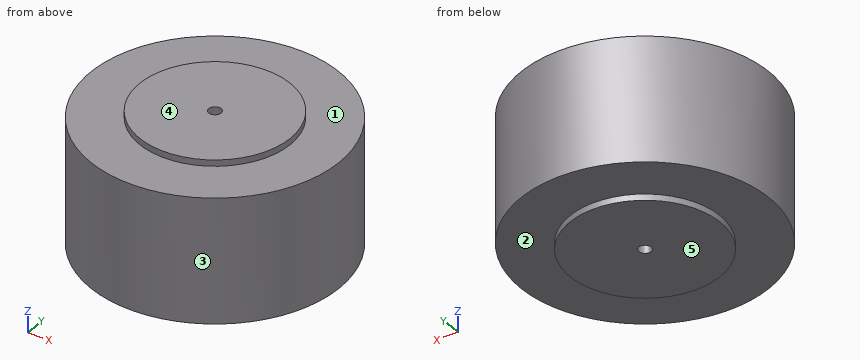
from build123d import *

# Parameters (mm, degrees)
SKETCH1_R           = 12.7
BOSS_EXTRUDE1_DEPTH = 12.7
SKETCH2_R           = 7.70834565
BOSS_EXTRUDE2_DEPTH = 0.635
SKETCH3_R           = 7.677981209
BOSS_EXTRUDE3_DEPTH = 0.635
SKETCH4_R           = 0.635
CUT_EXTRUDE1_DEPTH  = 1.27
SKETCH5_R           = 0.635
CUT_EXTRUDE2_DEPTH  = 1.27


with BuildPart() as part:
    # Sketch1 → Boss-Extrude1 (new body)
    with BuildSketch(Plane.XY):
        Circle(SKETCH1_R)
    extrude(amount=BOSS_EXTRUDE1_DEPTH)

    # Sketch2 → Boss-Extrude2 (add)
    with BuildSketch(Plane.XY.offset(12.7)):
        Circle(SKETCH2_R)
    extrude(amount=BOSS_EXTRUDE2_DEPTH)

    # Sketch3 → Boss-Extrude3 (add)
    with BuildSketch(Plane(origin=(0, 0, 0), x_dir=(-1, 0, 0), z_dir=(0, 0, -1))):
        Circle(SKETCH3_R)
    extrude(amount=BOSS_EXTRUDE3_DEPTH)

    # Sketch4 → Cut-Extrude1 (cut)
    with BuildSketch(Plane.XY.offset(13.335)):
        Circle(SKETCH4_R)
    extrude(amount=-CUT_EXTRUDE1_DEPTH, mode=Mode.SUBTRACT)

    # Sketch5 → Cut-Extrude2 (cut)
    with BuildSketch(Plane(origin=(0, 0, -0.635), x_dir=(-1, 0, 0), z_dir=(0, 0, -1))):
        Circle(SKETCH5_R)
    extrude(amount=-CUT_EXTRUDE2_DEPTH, mode=Mode.SUBTRACT)


solid = part.part
Here's how the part is built. I have some questions about the finished solid (model axes, mm). Face numbers are marked on the shaded views. A direction names the side the tool comes from. Round coordinates to 2 decimals unless told otherwise and drop trailing zeros. Write each loop counter-clockwise with the first axis right and the second up, starting at its lowest first coordinate (ties: lowest second). Pieces come first, ordered by that corner, then holes.
1. For the marked faces 1 and 2, which set-ups out of +Z, -Z, +X, -X, +Y, -Y let a thin tool reach every point of the face, with its end or its side?
2. I need wall thicknesses on L1, parallel to Y at x = 0, z = 12.65 (3 decimals); L2, parallel to Y at x = 0, z = -0.05 (3 decimals); L3, parallel to Z at x = 1.5, y = 11.25. Which ranges of each line are inside material? Lowest first, please.
3. Will these pins go through, and if not, where does the flat tip stop? pin 1 Ø3 at (x, z) = (-8.5, 9) entering from +Y; pin 2 Ø2 at (y, z) = (-5.5, 11.5) entering from +X; pin 3 Ø1.1 at (x, y) = (0, 0) entering from -Z (3 decimals).
4. Suppose I cut it at A-A (x = 0). List the corners of the cut face in (y, z) for me (3 decimals), and give its area (3 significant figures).
5. If we mould it in two halves opening along Z, with no side actions, what happens to the marked faces 3, 4 and 5? For each: released by +Z, released by -Z, zero draft, split by the parting line, or undercut.
6. Suppose I cut it at C-C (z = 2.5). List the corners of the cut face in (x, y) for me.
7. Suppose I cut it at D-D (x = -4.75). List the corners of the cut face in (y, z) for me (3 decimals).
Answer sheet:
1. face 1: +Z
1. face 2: -Z
2. L1: y = -12.7 to -0.635, 0.635 to 12.7
2. L2: y = -7.678 to -0.635, 0.635 to 7.678
2. L3: z = 0 to 12.7
3. pin 1: stops at y = 10.6
3. pin 2: stops at x = 11.88
3. pin 3: stops at z = 0.635
4. outline: (-12.7, 0) - (-7.678, 0) - (-7.678, -0.635) - (-0.635, -0.635) - (-0.635, 0.635) - (0.635, 0.635) - (0.635, -0.635) - (7.678, -0.635) - (7.678, 0) - (12.7, 0) - (12.7, 12.7) - (7.708, 12.7) - (7.708, 13.335) - (0.635, 13.335) - (0.635, 12.065) - (-0.635, 12.065) - (-0.635, 13.335) - (-7.708, 13.335) - (-7.708, 12.7) - (-12.7, 12.7) - close
4. area: 339 mm2
5. face 3: zero draft
5. face 4: released by +Z
5. face 5: released by -Z
6. outline: circle Ø25.4 at (0, 0)
7. outline: (-11.778, 0) - (-6.032, 0) - (-6.032, -0.635) - (6.032, -0.635) - (6.032, 0) - (11.778, 0) - (11.778, 12.7) - (6.071, 12.7) - (6.071, 13.335) - (-6.071, 13.335) - (-6.071, 12.7) - (-11.778, 12.7) - close
